from build123d import *

# Parameters (mm, degrees)
BOSS_EXTRUDE1_DEPTH = 6.35
SKETCH3_W           = 203.2
SKETCH3_H           = 12.7
BOSS_EXTRUDE2_DEPTH = 76.2
CAVITY1_START       = -6.35
CAVITY1_OUTLINE_R   = 12.7
CAVITY1_DEPTH       = 12.7


# Read off the part's stored shape, not the designer's step: Cavity1
with BuildPart() as part:
    # Sketch1 → Boss-Extrude1 (new, symmetric)
    with BuildSketch(Plane.XY):
        Polygon((732.36, 381), (785.7, 381), (1001.6, 381), (1087.96, 381), (1087.96, 685.8), (1001.6, 685.8), (785.7, 685.8), (732.36, 685.8), align=None)
    extrude(amount=BOSS_EXTRUDE1_DEPTH, both=True)

    # Sketch3 → Boss-Extrude2 (add)
    with BuildSketch(Plane.XZ.offset(-381)):
        with Locations((910.16, 0)):
            Rectangle(SKETCH3_W, SKETCH3_H)
    extrude(amount=BOSS_EXTRUDE2_DEPTH)

    # Cavity1 outline → Cavity1 (cut)
    with BuildSketch(Plane.XY.offset(CAVITY1_START)):
        with Locations((910.16, 546.1)):
            Circle(CAVITY1_OUTLINE_R)
    extrude(amount=CAVITY1_DEPTH, mode=Mode.SUBTRACT)


solid = part.part
Input: part model. Units: mm. Frame: model coordinates. A direction names the side the tool comes from. Give positions to 0.01 mm unless a question says otherwise; leave off trailing zeros. Loops run counter-clockwise (first coordinate to the right, second up) from the corner with the lowest first, then second, coordinate; pieces in that order, holes last. Notation, with made-up numbers: (89.5, 6) -> (97.5, 6) arc R24 cw to (97.5, 32) -> close; hole circle Ø4 at (20.5, 64.5). An arc over 180 degrees is marked (long way). Answer as a JSON object with one key per item and string values. Group by question number.
Item 1: Reachability of faces 4 (the flat face through (909, 304.8, 0)), 5 (the flat face through (770, 381, 0)), 6 (the flat face through (1011.76, 343, 0)) from +Z, -Z, +X, -X, +Y, -Y: full face, straight path, thin tool, end or side. Return the list, or none.
Item 2: Cut plane B-B, the plane z = -4.25. Return the cut outline in (x, y).
Item 3: Pull-direction query (Y, two-part tool) for faces 1 (the flat face through (1049, 381, 0)), 2 (the flat face through (1087.96, 531, 0)), 3 (the cylindrical face through (897.472, 546.658, -0.089)); classes: released by +Y, released by -Y, zero draft, split by the parting line, or undercut.
Item 4: Cut plane C-C, the plane y = 546.1. Return the cut outline in (x, z).
Item 5: Cut plane D-D, the plane y = 336. Return the cut outline in (x, z), and give its area (3 significant figures).
Item 6: Line query: probe 1 along X at (y, z) = (546.1, 3); probe 2 along Y at (x, z) = (910.16, -0.5); probe 3 along Y at (x, z) = (787.5, 3). Output: solid intervals per line, ascending.
Item 7: Pin query (flat end, axial travel): P1, Ø4, axis at x = 1064.5, z = -0.5, coming from the -Y side; P2, Ø6.5, axis at y = 336, z = 2.5, coming from the +X side; P3, Ø4, axis at y = 335.5, z = -2.5, coming from the -X side; P4, Ø15, axis at x = 910.16, y = 546.1, coming from the -Z side. Return the tip coordinate at first contact, or that it passes through.
Item 8: Cut plane A-A, the plane x = 910.16. Return the cut outline in (y, z).
Checks:
{
 "1": {"face 4": "+Z, -Z, +X, -X, -Y", "face 5": "+Z, -Z, -X, -Y", "face 6": "+Z, -Z, +X, -Y"},
 "2": {"outline": "(732.36, 381) -> (808.56, 381) -> (808.56, 304.8) -> (1011.76, 304.8) -> (1011.76, 381) -> (1087.96, 381) -> (1087.96, 685.8) -> (732.36, 685.8) -> close; hole circle Ø25.4 at (910.16, 546.1)"},
 "3": {"face 1": "released by -Y", "face 2": "zero draft", "face 3": "undercut"},
 "4": {"outline": "(732.36, -6.35) -> (897.46, -6.35) -> (897.46, 6.35) -> (732.36, 6.35) -> close; (922.86, -6.35) -> (1087.96, -6.35) -> (1087.96, 6.35) -> (922.86, 6.35) -> close"},
 "5": {"outline": "(808.56, -6.35) -> (1011.76, -6.35) -> (1011.76, 6.35) -> (808.56, 6.35) -> close", "area": "2,580 mm²"},
 "6": {"probe 1": "x = 732.36 to 897.46, 922.86 to 1087.96", "probe 2": "y = 304.8 to 533.4, 558.8 to 685.8", "probe 3": "y = 381 to 685.8"},
 "7": {"P1": "stops at y = 381", "P2": "stops at x = 1011.76", "P3": "stops at x = 808.56", "P4": "passes through"},
 "8": {"outline": "(304.8, -6.35) -> (533.4, -6.35) -> (533.4, 6.35) -> (304.8, 6.35) -> close; (558.8, -6.35) -> (685.8, -6.35) -> (685.8, 6.35) -> (558.8, 6.35) -> close"}
}
